from build123d import *

# Parameters (mm, degrees)
F1_DEPTH = 2
F2_DEPTH = 10
F3_DEPTH = 11
F4_R     = 2.5


with BuildPart() as f1:
    # F0 (on Top) → F1 (new body)
    with BuildSketch(Plane.XY):
        with BuildLine():
            ThreePointArc((0, 2.5), (0.732233047, 0.732233047), (2.5, 0))
            Line((2.5, 0), (88.5, 0))
            ThreePointArc((88.5, 0), (90.267766953, 0.732233047), (91, 2.5))
            Line((91, 2.5), (91, 59.5))
            ThreePointArc((91, 59.5), (90.267766953, 61.267766953), (88.5, 62))
            Line((88.5, 62), (2.5, 62))
            ThreePointArc((2.5, 62), (0.732233047, 61.267766953), (0, 59.5))
            Line((0, 59.5), (0, 2.5))
        make_face()
        with BuildLine():
            Line((2, 2.5), (2, 59.5))
            ThreePointArc((2, 59.5), (2.1464466094, 59.8535533906), (2.5, 60))
            Line((2.5, 60), (88.5, 60))
            ThreePointArc((88.5, 60), (88.8535533906, 59.8535533906), (89, 59.5))
            Line((89, 59.5), (89, 2.5))
            ThreePointArc((89, 2.5), (88.8535533906, 2.1464466094), (88.5, 2))
            Line((88.5, 2), (2.5, 2))
            ThreePointArc((2.5, 2), (2.1464466094, 2.1464466094), (2, 2.5))
        make_face(mode=Mode.SUBTRACT)
        with BuildLine():
            ThreePointArc((2.5, 60), (2.1464466094, 59.8535533906), (2, 59.5))
            Line((2, 59.5), (2, 2.5))
            ThreePointArc((2, 2.5), (2.1464466094, 2.1464466094), (2.5, 2))
            Line((2.5, 2), (88.5, 2))
            ThreePointArc((88.5, 2), (88.8535533906, 2.1464466094), (89, 2.5))
            Line((89, 2.5), (89, 59.5))
            ThreePointArc((89, 59.5), (88.8535533906, 59.8535533906), (88.5, 60))
            Line((88.5, 60), (2.5, 60))
        make_face()
        with BuildLine():
            Line((3.5, 59), (87.5, 59))
            ThreePointArc((87.5, 59), (87.8535533906, 58.8535533906), (88, 58.5))
            Line((88, 58.5), (88, 3.5))
            ThreePointArc((88, 3.5), (87.8535533906, 3.1464466094), (87.5, 3))
            Line((87.5, 3), (3.5, 3))
            ThreePointArc((3.5, 3), (3.1464466094, 3.1464466094), (3, 3.5))
            Line((3, 3.5), (3, 58.5))
            ThreePointArc((3, 58.5), (3.1464466094, 58.8535533906), (3.5, 59))
        make_face(mode=Mode.SUBTRACT)
        with BuildLine():
            ThreePointArc((88, 58.5), (87.8535533906, 58.8535533906), (87.5, 59))
            Line((87.5, 59), (3.5, 59))
            ThreePointArc((3.5, 59), (3.1464466094, 58.8535533906), (3, 58.5))
            Line((3, 58.5), (3, 3.5))
            ThreePointArc((3, 3.5), (3.1464466094, 3.1464466094), (3.5, 3))
            Line((3.5, 3), (87.5, 3))
            ThreePointArc((87.5, 3), (87.8535533906, 3.1464466094), (88, 3.5))
            Line((88, 3.5), (88, 58.5))
        make_face()
    extrude(amount=F1_DEPTH)

    # F0 (on Top) → F2 (join)
    with BuildSketch(Plane.XY):
        with BuildLine():
            ThreePointArc((0, 2.5), (0.732233047, 0.732233047), (2.5, 0))
            Line((2.5, 0), (88.5, 0))
            ThreePointArc((88.5, 0), (90.267766953, 0.732233047), (91, 2.5))
            Line((91, 2.5), (91, 59.5))
            ThreePointArc((91, 59.5), (90.267766953, 61.267766953), (88.5, 62))
            Line((88.5, 62), (2.5, 62))
            ThreePointArc((2.5, 62), (0.732233047, 61.267766953), (0, 59.5))
            Line((0, 59.5), (0, 2.5))
        make_face()
        with BuildLine():
            Line((2, 2.5), (2, 59.5))
            ThreePointArc((2, 59.5), (2.1464466094, 59.8535533906), (2.5, 60))
            Line((2.5, 60), (88.5, 60))
            ThreePointArc((88.5, 60), (88.8535533906, 59.8535533906), (89, 59.5))
            Line((89, 59.5), (89, 2.5))
            ThreePointArc((89, 2.5), (88.8535533906, 2.1464466094), (88.5, 2))
            Line((88.5, 2), (2.5, 2))
            ThreePointArc((2.5, 2), (2.1464466094, 2.1464466094), (2, 2.5))
        make_face(mode=Mode.SUBTRACT)
    extrude(amount=F2_DEPTH)

    # F0 (on Top) → F3 (join)
    with BuildSketch(Plane.XY):
        with BuildLine():
            ThreePointArc((2.5, 60), (2.1464466094, 59.8535533906), (2, 59.5))
            Line((2, 59.5), (2, 2.5))
            ThreePointArc((2, 2.5), (2.1464466094, 2.1464466094), (2.5, 2))
            Line((2.5, 2), (88.5, 2))
            ThreePointArc((88.5, 2), (88.8535533906, 2.1464466094), (89, 2.5))
            Line((89, 2.5), (89, 59.5))
            ThreePointArc((89, 59.5), (88.8535533906, 59.8535533906), (88.5, 60))
            Line((88.5, 60), (2.5, 60))
        make_face()
        with BuildLine():
            Line((3.5, 59), (87.5, 59))
            ThreePointArc((87.5, 59), (87.8535533906, 58.8535533906), (88, 58.5))
            Line((88, 58.5), (88, 3.5))
            ThreePointArc((88, 3.5), (87.8535533906, 3.1464466094), (87.5, 3))
            Line((87.5, 3), (3.5, 3))
            ThreePointArc((3.5, 3), (3.1464466094, 3.1464466094), (3, 3.5))
            Line((3, 3.5), (3, 58.5))
            ThreePointArc((3, 58.5), (3.1464466094, 58.8535533906), (3.5, 59))
        make_face(mode=Mode.SUBTRACT)
    extrude(amount=F3_DEPTH)

    # F4
    f4_edges = [f1.edges().sort_by_distance(p)[0] for p in [
        (45.5, 0, 0),
    ]]
    fillet(f4_edges, radius=F4_R)


solid = f1.part
For this review, take the finished solid that the model builds, in its own axes (mm). A direction names the side the tool comes from. Coordinates: 2 decimals unless noted, no trailing zeros. Order: outer loops, then holes, each group sorted by start corner. A loop starts at its lowest first (then second) coordinate and runs counter-clockwise, first axis right, second up. Notation, with made-up numbers: (49.5, -22.5) - (60.5, -22.5) arc R23 ccw to (60.5, -9.5) - close; hole circle Ø10 at (45.5, -30.5). An arc over 180 degrees is marked (long way). Answer as CSV lines item,"result". Start each with the question number.
1) To check wall thickness, follow line 1 along Y through (x, z) = (15, 5); line 2 along Y through (x, z) = (42.5, 10.5); line 3 along X through (y, z) = (22.5, 8.75). State the ranges of each line that lie inside material, in increasing order. Write a range as [from, to].
2) Add section A-A (z = 9). State the section outline as (x, y) points.
3) Insertion check: P1, Ø8, axis at x = 58, y = 52.5, coming from the +Z side; P2, Ø0.8, axis at x = 29.5, z = 10.5, coming from the +Y side; P3, Ø4, axis at x = 29.5, z = 2, coming from the +Y side; P4, Ø0.5, axis at y = 17, z = 10.5, coming from the -X side. Each pin has a flat end and moves straight along its axis. Give the tip position at first contact, or say it passes through.
4) Add section B-B (y = 17). State the section outline as (x, z) points.
5) Draft analysis for pull direction X (two halves, no side actions). For faces 3 (the flat face through (45, 31, 0)), 4 (the flat face through (88, 31, 6)), 5 (the cylindrical face through (90.248, 0.713, 6.198)), 6 (the flat face through (45, 31, 2)), state which applies: +X half, -X half, draft (parallel to the pull), parting line (faces both ways), or undercut.
6) Machinability: for faces 1 (the cylindrical face through (44.898, 61.248, 0.713)), 2 (the flat face through (46, 3, 6)), which of the approach directions +Z, -Z, +X, -X, +Y, -Y give a long, thin tool a straight path to every point of the face, cutting with its end or side? Answer none if there is none.
7) Add section C-C (x = 73). State the section outline as (y, z) points.
Result:
1,line 1,"[0, 3], [59, 62]"
1,line 2,"[2, 3], [59, 60]"
1,line 3,"[0, 3], [88, 91]"
2,outline,"(0, 2.5) arc R2.5 ccw to (2.5, 0) - (88.5, 0) arc R2.5 ccw to (91, 2.5) - (91, 59.5) arc R2.5 ccw to (88.5, 62) - (2.5, 62) arc R2.5 ccw to (0, 59.5) - close; hole (3, 3.5) arc R0.5 ccw to (3.5, 3) - (87.5, 3) arc R0.5 ccw to (88, 3.5) - (88, 58.5) arc R0.5 ccw to (87.5, 59) - (3.5, 59) arc R0.5 ccw to (3, 58.5) - close"
3,P1,"z = 2"
3,P2,"y = 60"
3,P3,"y = 62"
3,P4,"x = 2"
4,outline,"(0, 2.5) arc R2.5 ccw to (2.5, 0) - (88.5, 0) arc R2.5 ccw to (91, 2.5) - (91, 10) - (89, 10) - (89, 11) - (88, 11) - (88, 2) - (3, 2) - (3, 11) - (2, 11) - (2, 10) - (0, 10) - close"
5,face 3,"draft"
5,face 4,"undercut"
5,face 5,"+X half"
5,face 6,"undercut"
6,face 1,"-Z, +X, -X, +Y"
6,face 2,"+Z"
7,outline,"(0, 2.5) arc R2.5 ccw to (2.5, 0) - (59.5, 0) arc R2.5 ccw to (62, 2.5) - (62, 10) - (60, 10) - (60, 11) - (59, 11) - (59, 2) - (3, 2) - (3, 11) - (2, 11) - (2, 10) - (0, 10) - close"
